Source: three-view drawing plus pictorial views. Frame: mm from the lowest corner of the part. A direction names the side the tool comes from. Coordinates: 2 decimals unless noted, no trailing zeros. Write each loop counter-clockwise with the first axis right and the second up, starting at its lowest first coordinate (ties: lowest second). Pieces come first, ordered by that corner, then holes. Notation, with made-up numbers: (19.5, 56.5) -> (31.5, 56.5) arc R17 cw to (31.5, 73.5) -> close; hole circle Ø8 at (71.5, 59.5). An arc over 180 degrees is marked (long way). One line per item, written item: value.
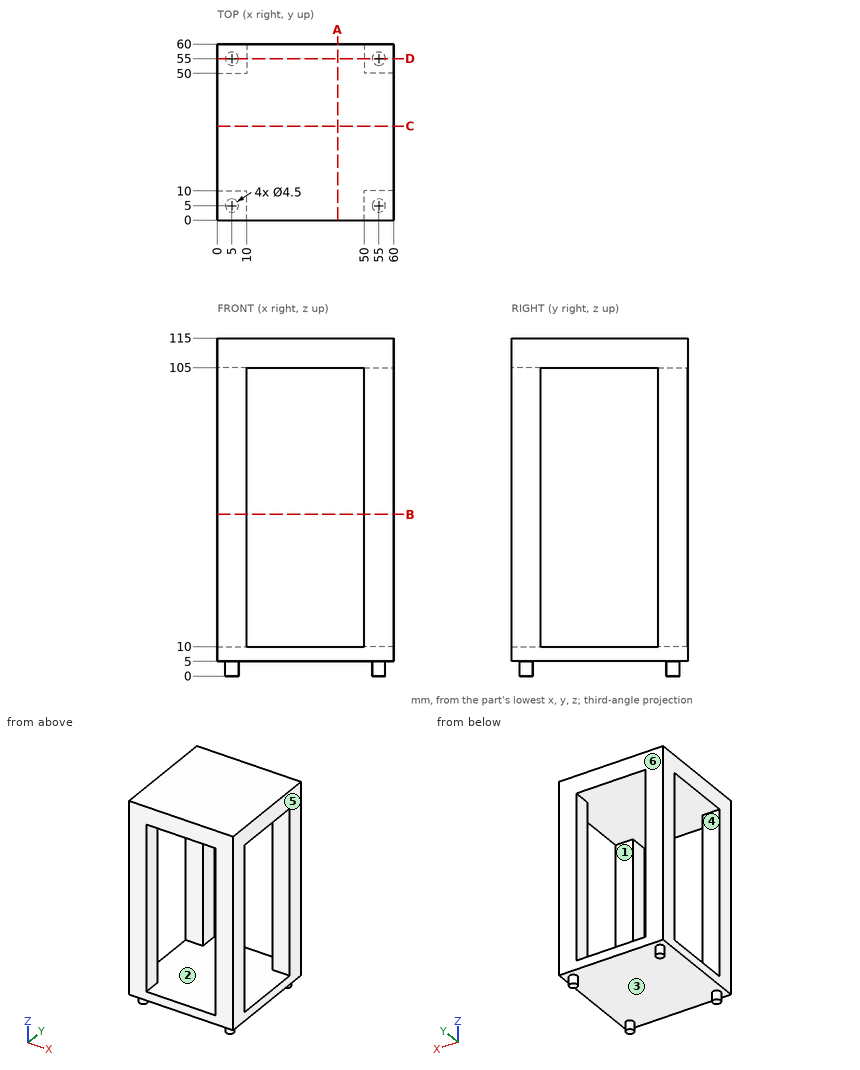
(1) Pull-direction query (Y, two-part tool) for the marked faces 4, 5 and 6; classes: released by +Y, released by -Y, zero draft, split by the parting line, or undercut.
Responses:
face 4: undercut
face 5: zero draft
face 6: released by +Y
(2) Section A-A (x = 41). Return the cut outline in (y, z), then the cut area to 3 significant figures.
Responses:
outline: (0, 5) -> (60, 5) -> (60, 10) -> (0, 10) -> close; (0, 105) -> (60, 105) -> (60, 115) -> (0, 115) -> close
area: 900 mm2
(3) Reachability of the marked faces 1, 2 and 3 from +Z, -Z, +X, -X, +Y, -Y: full face, straight path, thin tool, end or side. Return the list, or none.
Responses:
face 1: +X, -X
face 2: none
face 3: -Z
(4) Section D-D (y = 55). Return the cut outline in (x, z).
Responses:
outline: (0, 5) -> (2.75, 5) -> (2.75, 0) -> (7.25, 0) -> (7.25, 5) -> (52.75, 5) -> (52.75, 0) -> (57.25, 0) -> (57.25, 5) -> (60, 5) -> (60, 115) -> (0, 115) -> close; hole (10, 10) -> (50, 10) -> (50, 105) -> (10, 105) -> close
(5) Line query: line 1 (Y direction, x = 2, z = 52); line 2 (Z direction, x = 29.5, y = 45). Output: solid intervals per line, ascending. Write a range as [from, to].
Responses:
line 1: y = [0, 10], [50, 60]
line 2: z = [5, 10], [105, 115]
(6) Section B-B (z = 55). Return the cut outline in (x, y), then the cut area to 3 significant figures.
Responses:
outline: (0, 0) -> (10, 0) -> (10, 10) -> (0, 10) -> close; (0, 50) -> (10, 50) -> (10, 60) -> (0, 60) -> close; (50, 0) -> (60, 0) -> (60, 10) -> (50, 10) -> close; (50, 50) -> (60, 50) -> (60, 60) -> (50, 60) -> close
area: 400 mm2
(7) First-contact query: pin 1 (18 mm diameter, centred on x = 16.5, y = 35.5, fed in from -Z). Flat tip, straight axial feed; report the tip coordinate or a pass-through.
Responses:
pin 1: stops at z = 5
